The figure shows three views and two pictorial views of one solid part (mm, origin at its lowest corner). Answer the questions. A direction names the side the tool comes from. Give positions to 0.01 mm unless a question says otherwise; leave off trailing zeros. Loops run counter-clockwise (first coordinate to the right, second up) from the corner with the lowest first, then second, coordinate; pieces in that order, holes last. Notation, with made-up numbers: M 59.5,10 L 70.5,10 A22 ccw 70.5,34 Z; hole C 18,-36.5 d10. An arc over 180 degrees is marked long. Answer in a Markdown table with one row per item. Add a question column.
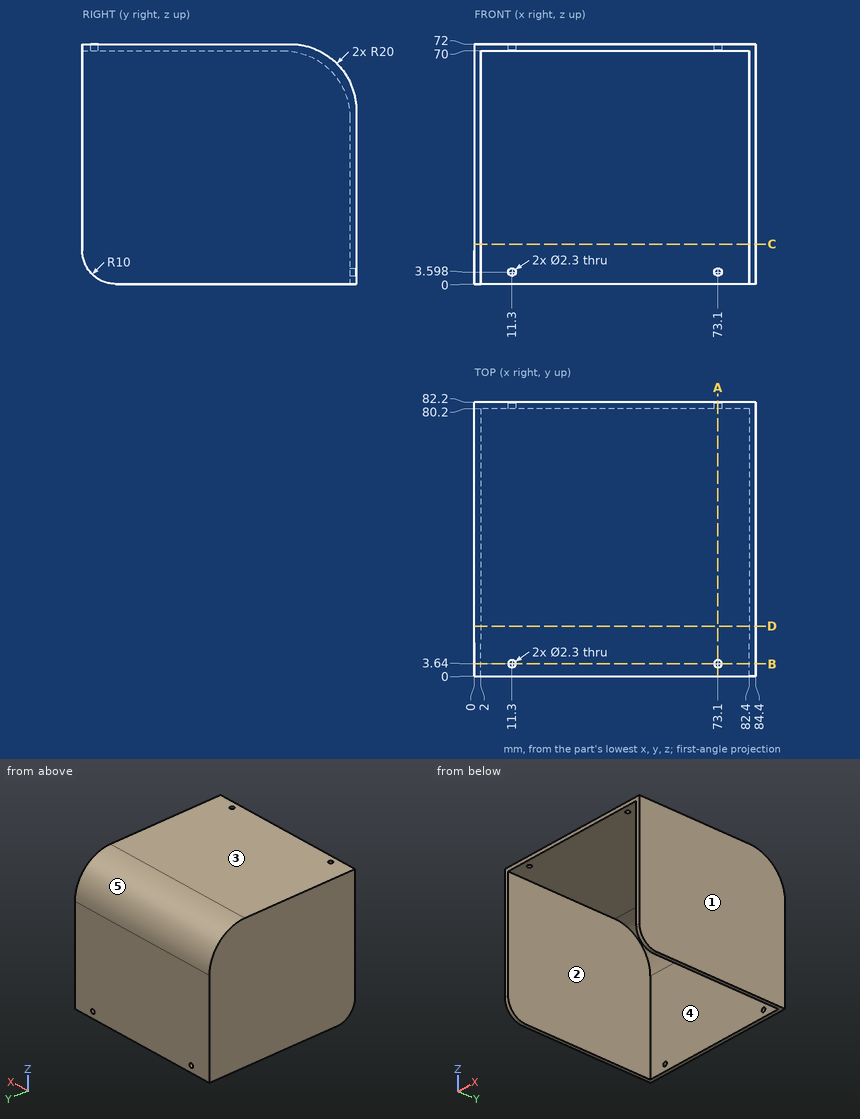
(1) Section B-B, the plane y = 3.64 is taken. Determine the outline of the cut face in (x, z), and give its area (3 significant figures).
(2) Each of these flat-tipped pins is pushed along its axis until it touches: P1, Ø1.4, axis at x = 73.1, z = 3.6, coming from the +Y side (1 decimal); P2, Ø4, axis at x = 51.5, y = 74, coming from the +Z side; P3, Ø2.5, axis at x = 11.3, z = 3.6, coming from the -Y side. Where does it stop, or does it pass through?
(3) The mould has two halves that part along X. Classify the marked faces 1, 2 and 3: pulls with the +X half, pulls with the -X half, needs draft (parallel to the pull), parting line crosses it, or undercut.
(4) Section A-A, the plane x = 73.1 is taken. Determine the outline of the cut face in (y, z).
(5) Consider line 1 along X through (y, z) = (67, 39.5); line 2 along Y through (x, z) = (65, 9); line 3 along Z through (x, y) = (10.5, 48.5). Determine where each line is inside the solid, lowest interval first. Write a range as from..to.
(6) Section C-C, the plane z = 12 is taken. Determine the outline of the cut face in (x, y), and give its area (3 significant figures).
(7) Section D-D, the plane y = 15 is taken. Determine the outline of the cut face in (x, z), and give its area (3 significant figures).
(8) Which of the six approach directions +Z, -Z, +X, -X, +Y, -Y give full straight-line access (tool end or side, diameter ignored) to the marked faces 4 and 5?
Numbers:
| question | item | result |
|---|---|---|
| 1 | outline | M 0,2.28 L 2,2.28 L 2,70 L 10.15,70 L 10.15,72 L 0,72 Z; M 12.45,70 L 71.95,70 L 71.95,72 L 12.45,72 Z; M 74.25,70 L 82.4,70 L 82.4,2.28 L 84.4,2.28 L 84.4,72 L 74.25,72 Z |
| 1 | area | 430 mm² |
| 2 | P1 | passes through |
| 2 | P2 | stops at z = 69.43 |
| 2 | P3 | stops at y = 80.2 |
| 3 | face 1 | pulls with the +X half |
| 3 | face 2 | undercut |
| 3 | face 3 | needs draft |
| 4 | outline | M 0,70 L 2.49,70 L 2.49,72 L 0,72 Z; M 4.79,70 L 60.2,70 A20 cw 80.2,50 L 80.2,4.75 L 82.2,4.75 L 82.2,52 A20 ccw 62.2,72 L 4.79,72 Z; M 80.2,0 L 82.2,0 L 82.2,2.45 L 80.2,2.45 Z |
| 5 | line 1 | x = 0..2, 82.4..84.4 |
| 5 | line 2 | y = 80.2..82.2 |
| 5 | line 3 | z = 70..72 |
| 6 | outline | M 0,0 L 2,0 L 2,80.2 L 82.4,80.2 L 82.4,0 L 84.4,0 L 84.4,82.2 L 0,82.2 Z |
| 6 | area | 490 mm² |
| 7 | outline | M 0,0 L 2,0 L 2,70 L 82.4,70 L 82.4,0 L 84.4,0 L 84.4,72 L 0,72 Z |
| 7 | area | 449 mm² |
| 8 | face 4 | -Z, -Y |
| 8 | face 5 | +Z, +X, -X, +Y |
